Geometry check sheet. Reference: the model listing, model coordinates, mm. Face numbers are marked on the shaded views. Round coordinates to 2 decimals unless told otherwise and drop trailing zeros. Order: outer loops, then holes, each group sorted by start corner. A loop starts at its lowest first (then second) coordinate and runs counter-clockwise, first axis right, second up. Notation, with made-up numbers: (-32, -30) - (-10, -30) arc R14 cw to (-10, -18) - close; hole circle Ø3 at (44, -26.75). An arc over 180 degrees is marked (long way). Return JSON: item names as keys, results as strings. Group by question number.
Q1. Sectioned sample at C-C, the plane z = 0. Record the cut outline in (x, y).
Q2. Sectioned sample at B-B, the plane y = -7. Record the cut outline in (x, z).
Q3. Material ranges on line 1 along Z through (x, y) = (0, -8.15); line 2 along Z through (x, y) = (37.5, -0.25); line 3 along Y through (x, z) = (-31.5, -43), recorded low to high.
Q4. Gauge pin test, flat ends, axial feed: pin 1 Ø5.5 at (x, y) = (-1, -8.5) entering from -Z; pin 2 Ø4 at (y, z) = (-8, 2) entering from -X; pin 3 Ø11.5 at (x, z) = (0, 0) entering from +Y. Record the tip position at first contact, or that the pin passes through.
Q5. Draft check along Z on the marked faces 1 and 2. Enter one of: pulls with the +Z half, pulls with the -Z half, needs draft (parallel to the pull), parting line crosses it, or undercut.
Q6. Sectioned sample at A-A, the plane x = 0. Record the cut outline in (y, z).
Q7. Sectioned sample at D-D, the plane z = -37. Record the cut outline in (x, y).
```python
from build123d import *

# Parameters (mm, degrees)
F0_W     = 100
F0_H     = 100
F0_W_2   = 95
F0_H_2   = 95
F1_DEPTH = 5
F2_DEPTH = 2
F3_W     = 30
F3_H     = 30
F4_DEPTH = 5
F5_R     = 5
F6_DEPTH = 5


with BuildPart() as f1:
    # F0 (on Front) → F1 (new body)
    with BuildSketch(Plane.XZ):
        Rectangle(F0_W, F0_H)
        Rectangle(F0_W_2, F0_H_2, mode=Mode.SUBTRACT)
        Rectangle(F0_W_2, F0_H_2)
    extrude(amount=F1_DEPTH)

    # F0 (on Front) → F2 (cut)
    with BuildSketch(Plane.XZ):
        Rectangle(F0_W_2, F0_H_2)
    extrude(amount=F2_DEPTH, mode=Mode.SUBTRACT)

    # F3 (on face) → F4 (join)
    with BuildSketch(Plane.XZ.offset(5)):
        Rectangle(F3_W, F3_H)
    extrude(amount=F4_DEPTH)

    # F5 (on face) → F6 (cut)
    with BuildSketch(Plane.XZ.offset(10)):
        Circle(F5_R)
    extrude(amount=-F6_DEPTH, mode=Mode.SUBTRACT)


solid = f1.part
```
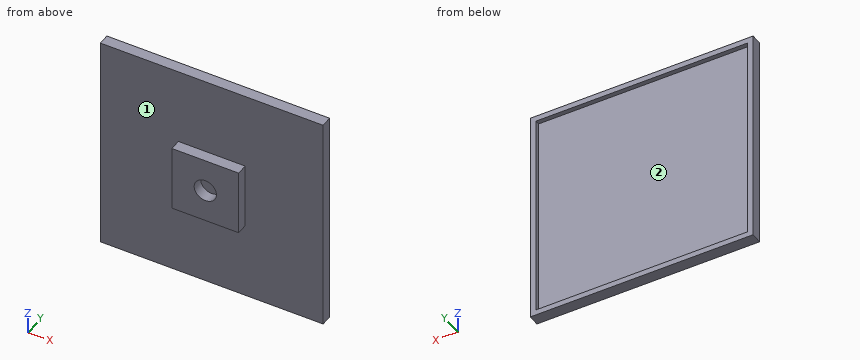
Reply:
{
 "1": {"outline": "(-50, -5) - (-15, -5) - (-15, -10) - (-5, -10) - (-5, -5) - (5, -5) - (5, -10) - (15, -10) - (15, -5) - (50, -5) - (50, 0) - (47.5, 0) - (47.5, -2) - (-47.5, -2) - (-47.5, 0) - (-50, 0) - close"},
 "2": {"outline": "(-15, -15) - (15, -15) - (15, 15) - (-15, 15) - close; hole circle Ø10 at (0, 0)"},
 "3": {"line 1": "-15 to -5, 5 to 15", "line 2": "-50 to -47.5, 47.5 to 50", "line 3": "-5 to -2"},
 "4": {"pin 1": "z = -15", "pin 2": "x = -15", "pin 3": "y = -2"},
 "5": {"face 1": "needs draft", "face 2": "undercut"},
 "6": {"outline": "(-10, -15) - (-5, -15) - (-5, -50) - (0, -50) - (0, -47.5) - (-2, -47.5) - (-2, 47.5) - (0, 47.5) - (0, 50) - (-5, 50) - (-5, 15) - (-10, 15) - (-10, 5) - (-5, 5) - (-5, -5) - (-10, -5) - close"},
 "7": {"outline": "(-50, -5) - (50, -5) - (50, 0) - (47.5, 0) - (47.5, -2) - (-47.5, -2) - (-47.5, 0) - (-50, 0) - close"}
}
